Check sheet for the modelled part. Datum: model origin and axes. Units: mm. A direction names the side the tool comes from. Coordinates: 2 decimals unless noted, no trailing zeros. Loops run counter-clockwise (first coordinate to the right, second up) from the corner with the lowest first, then second, coordinate; pieces in that order, holes last.
```python
from build123d import *

# Parameters (mm, degrees)
SZKIC1_W                    = 13
SZKIC1_H                    = 7.5
DODANIE_WYCI_GNI_CIE1_DEPTH = 3
SZKIC2_W                    = 11
SZKIC2_H                    = 3.5
WYTNIJ_WYCI_GNI_CIE1_DEPTH  = 3
ZAOKR_GLENIE1_R             = 3
SZKIC3_R                    = 3
SZKIC3_R_2                  = 2
DODANIE_WYCI_GNI_CIE2_DEPTH = 3
WYTNIJ_WYCI_GNI_CIE2_DEPTH  = 3
ZAOKR_GLENIE2_R             = 0.3


with BuildPart() as part:
    # Szkic1 → Dodanie-wyciągnięcie1 (new body)
    with BuildSketch(Plane.XY):
        with Locations((6.5, 3.75)):
            Rectangle(SZKIC1_W, SZKIC1_H)
    extrude(amount=DODANIE_WYCI_GNI_CIE1_DEPTH)

    # Szkic2 → Wytnij-wyciągnięcie1 (cut)
    with BuildSketch(Plane.XY.offset(3)):
        with Locations((5.5, 3.75)):
            Rectangle(SZKIC2_W, SZKIC2_H)
    extrude(amount=-WYTNIJ_WYCI_GNI_CIE1_DEPTH, mode=Mode.SUBTRACT)

    # Zaokrąglenie1
    # the kernel refuses this fillet: 3 mm, written as the material it takes off along each edge
    with BuildSketch(Plane(origin=(13, 7.5, -7.5), x_dir=(0, -1, 0), z_dir=(0, 0, 1))) as zaokr_glenie1_piece_1:
        with BuildLine():
            CenterArc((ZAOKR_GLENIE1_R, -ZAOKR_GLENIE1_R), ZAOKR_GLENIE1_R, 90, 90)
            Line((0, -ZAOKR_GLENIE1_R), (-ZAOKR_GLENIE1_R * 0.02, -ZAOKR_GLENIE1_R))
            Line((-ZAOKR_GLENIE1_R * 0.02, -ZAOKR_GLENIE1_R), (-ZAOKR_GLENIE1_R * 0.02, ZAOKR_GLENIE1_R * 0.02))
            Line((-ZAOKR_GLENIE1_R * 0.02, ZAOKR_GLENIE1_R * 0.02), (ZAOKR_GLENIE1_R, ZAOKR_GLENIE1_R * 0.02))
            Line((ZAOKR_GLENIE1_R, ZAOKR_GLENIE1_R * 0.02), (ZAOKR_GLENIE1_R, 0))
        make_face()
    extrude(amount=18, mode=Mode.SUBTRACT)
    with BuildSketch(Plane(origin=(0, 0, -7.071067812), x_dir=(1, 0, 0), z_dir=(0, 0, 1))) as zaokr_glenie1_piece_2:
        with BuildLine():
            CenterArc((2.828427125, 3), ZAOKR_GLENIE1_R, 199.471220634, 70.528779366)
            Line((0, 2), (-0.056568542, 1.98))
            ThreePointArc((-0.056568542, 1.98), (-0.06, 1), (-0.06, 0))
            Line((-0.06, 0), (0, -0.06))
            Line((0, -0.06), (2.828427125, -0.06))
            Line((2.828427125, -0.06), (2.828427125, 0))
        make_face()
    extrude(amount=17.142135624, mode=Mode.SUBTRACT)
    with BuildSketch(Plane(origin=(0, 7.5, -7.071067812), x_dir=(1, 0, 0), z_dir=(0, 0, 1))) as zaokr_glenie1_piece_3:
        with BuildLine():
            CenterArc((2.828427125, -3), ZAOKR_GLENIE1_R, 90, 70.528779366)
            Line((0, -2), (-0.056568542, -1.98))
            ThreePointArc((-0.056568542, -1.98), (-0.06, -1), (-0.06, 0))
            Line((-0.06, 0), (0, 0.06))
            Line((0, 0.06), (2.828427125, 0.06))
            Line((2.828427125, 0.06), (2.828427125, 0))
        make_face()
    extrude(amount=17.142135624, mode=Mode.SUBTRACT)

    # Szkic3 → Dodanie-wyciągnięcie2 (add)
    with BuildSketch(Plane.XY.offset(3)):
        with Locations((10, -1.5)):
            Circle(SZKIC3_R)
        with Locations((10, -1.5)):
            Circle(SZKIC3_R_2, mode=Mode.SUBTRACT)
    extrude(amount=-DODANIE_WYCI_GNI_CIE2_DEPTH)

    # Szkic4 → Wytnij-wyciągnięcie2 (cut)
    with BuildSketch(Plane.XY.offset(3)):
        Polygon((10, 0), (13, 0), (13, -1.5), (10, -1.990922123), align=None)
    extrude(amount=-WYTNIJ_WYCI_GNI_CIE2_DEPTH, mode=Mode.SUBTRACT)

    # Zaokrąglenie2
    zaokr_glenie2_edges = [part.edges().sort_by_distance(p)[0] for p in [
        (0, 2, 1.5),
        (0, 5.5, 1.5),
        (13, -1.5, 1.5),
        (13, 0, 1.5),
    ]]
    fillet(zaokr_glenie2_edges, radius=ZAOKR_GLENIE2_R)


solid = part.part
```
1) Section check C-C on z = 1. Enter the section's corners in (x, y).
Answer sheet:
outline: (0.2, 1.56) arc R3 ccw to (2.83, 0) - (7.4, 0) arc R3 ccw (long way) to (12.97, -1.9) arc R0.3 ccw to (12.63, -1.56) - (11.99, -1.66) arc R2 cw (long way) to (8.68, 0) - (12.7, 0) arc R0.3 ccw to (13, 0.3) - (13, 4.5) arc R3 ccw to (10, 7.5) - (2.83, 7.5) arc R3 ccw to (0.2, 5.94) arc R0.3 ccw to (0.46, 5.5) - (11, 5.5) - (11, 2) - (0.46, 2) arc R0.3 ccw to start
2) Mould release check, pull along Y, two halves, no side actions. Record for faces 1 (the cylindrical face through (12.14, 6.6, 1.48)), 2 (the flat face through (6, 2, 2)), 3 (the flat face through (7.9, 1.6, 0)): +Y half, -Y half, draft (parallel to the pull), parting line (faces both ways), or undercut.
Answer sheet:
face 1: +Y half
face 2: undercut
face 3: draft
3) Depth check by flat-ended pin: pin 1 (0.9 mm diameter, centred on x = 5.5, z = 1.5, fed in from -Y); pin 2 (2 mm diameter, centred on x = 4.5, y = -1.5, fed in from +Z); pin 3 (1 mm diameter, centred on y = 1, z = 1, fed in from -X). Enter the tip coordinate at first touch or a pass-through.
Answer sheet:
pin 1: stops at y = 0
pin 2: passes through
pin 3: stops at x = 0.23
4) Set-up check for faces 4 (the flat face through (11, 0, 1)), 5 (the flat face through (6, 5.5, 2)), 6 (the cylindrical face through (1.32, 7.093, 1.479)): record each of +Z, -Z, +X, -X, +Y, -Y from which the full face is reachable in a straight line by a thin tool's end or side.
Answer sheet:
face 4: +Z, -Z, +X
face 5: +Z, -Z, -X
face 6: +Z, -Z, -X, +Y
5) Section check B-B on y = -3.25. Enter the section's corners in (x, z), plus the area to 3 significant figures.
Answer sheet:
outline: (7.56, 0) - (9.03, 0) - (9.03, 3) - (7.56, 3) - close; (10.97, 0) - (12.44, 0) - (12.44, 3) - (10.97, 3) - close
area: 8.81 mm2
6) Scan lines: line 1 (Y direction, x = 10, z = 1.95); line 2 (Y direction, x = 3.25, z = 1.9); line 3 (Y direction, x = 8.5, z = 2.6). Record each from-to range of solid material in increasing order.
Answer sheet:
line 1: y = -4.5 to -3.5, 0 to 2, 5.5 to 7.5
line 2: y = 0 to 2, 5.5 to 7.5
line 3: y = -4.1 to -2.82, -0.18 to 2, 5.5 to 7.5
7) Section check D-D on y = 2.25. Enter the section's corners in (x, z), plus the area to 3 significant figures.
Answer sheet:
outline: (11, 0) - (13, 0) - (13, 3) - (11, 3) - close
area: 6.00 mm2
8) Section check A-A on x = 6.5. Enter the section's corners in (y, z), plus the area to 3 significant figures.
Answer sheet:
outline: (0, 0) - (2, 0) - (2, 3) - (0, 3) - close; (5.5, 0) - (7.5, 0) - (7.5, 3) - (5.5, 3) - close
area: 12.0 mm2
